Part model, mm, in its own coordinate system. A direction names the side the tool comes from. Give positions to 0.01 mm unless a question says otherwise; leave off trailing zeros. Order: outer loops, then holes, each group sorted by start corner. A loop starts at its lowest first (then second) coordinate and runs counter-clockwise, first axis right, second up. Notation, with made-up numbers: M 89.25,-5 L 130.25,-5 A38 ccw 130.25,34 Z; hole C 10,-32.5 d1. An arc over 180 degrees is marked long. One line per question, with ' | ' between items.
Autodesk Inventor part; units mm, degrees
ref_plane "YZ Plane" through (0, 0, 0) normal (1, 0, 0) x (0, 1, 0)
ref_plane "XZ Plane" through (0, 0, 0) normal (0, 1, 0) x (-1, 0, 0)
ref_plane "XY Plane" through (0, 0, 0) normal (0, 0, 1) x (1, 0, 0)
sketch "스케치1" plane through (0, 0, 0) normal (0, 0, 1) x (1, 0, 0)
  line L0 (-22.5, -10.25) -> (22.5, -10.25)
  line L1 (22.5, -10.25) -> (22.5, 10.25)
  line L2 (22.5, 10.25) -> (-22.5, 10.25)
  line L3 (-22.5, 10.25) -> (-22.5, -10.25)
  line L4 (-22.5, -10.25) -> (22.5, 10.25) construction
  line L5 (22.5, -10.25) -> (-22.5, 10.25) construction
  point P0 (0, 0)
  dimension "d0" = 45
  dimension "d1" = 20.5
extrude "돌출1" add sketch "스케치1" along normal blind 1.2
sketch "스케치2" plane through (-22.5, -10.25, 0) normal (-1, 0, 0) x (0, 0, 1)
  line L0 (1.2, 0) -> (1.2, 20.5)
  line L1 (4.05, 6.65) -> (1.2, 6.65) construction
  line L2 (1.2, 6.65) -> (1.2, 13.85)
  line L3 (1.2, 13.85) -> (4.05, 13.85) construction
  line L4 (4.05, 13.2546) -> (4.05, 7.2454)
  line L5 (4.05, 6.65) -> (1.2, 13.85) construction
  line L6 (1.2, 6.65) -> (4.05, 13.85) construction
  line L7 (1.6136, 13.4226) -> (3.4636, 13.7471)
  line L8 (1.6136, 7.0774) -> (3.4636, 6.7529)
  line L9 (1.2, 12.9301) -> (1.2, 7.5699)
  line L10 (3.85, 7.4835) -> (3.85, 13.0165)
  line L11 (3.2636, 13.509) -> (1.8136, 13.2546)
  line L12 (1.4, 12.7621) -> (1.4, 7.7379)
  line L13 (1.8136, 7.2454) -> (3.2636, 6.991)
  line L14 (2.375, 8.25) -> (2.875, 8.25)
  line L15 (2.875, 8.25) -> (2.875, 12.25)
  line L16 (2.875, 12.25) -> (2.375, 12.25)
  line L17 (2.375, 12.25) -> (2.375, 8.25)
  line L18 (2.375, 8.25) -> (2.875, 12.25) construction
  line L19 (2.875, 8.25) -> (2.375, 12.25) construction
  arc A0 (1.6136, 13.4226) -> (1.2, 12.9301) centre (1.7, 12.9301) ccw
  arc A1 (4.05, 13.2546) -> (3.4636, 13.7471) centre (3.55, 13.2546) ccw
  arc A2 (3.4636, 6.7529) -> (4.05, 7.2454) centre (3.55, 7.2454) ccw
  arc A3 (1.2, 7.5699) -> (1.6136, 7.0774) centre (1.7, 7.5699) ccw
  arc A4 (1.4, 7.7379) -> (1.8136, 7.2454) centre (1.9, 7.7379) ccw
  arc A5 (3.2636, 6.991) -> (3.85, 7.4835) centre (3.35, 7.4835) ccw
  arc A6 (3.85, 13.0165) -> (3.2636, 13.509) centre (3.35, 13.0165) ccw
  arc A7 (1.8136, 13.2546) -> (1.4, 12.7621) centre (1.9, 12.7621) ccw
  point P0 (0, 10.25)
  point P1 (2.625, 10.25)
  point P2 (1.2, 10.25)
  point P3 (1.2, 13.35)
  point P4 (1.2, 7.15)
  dimension "d4" = 2.85
  dimension "d5" = 7.2
  dimension "d6" = 0.5
  dimension "d7" = 0.5
  dimension "d8" = 0.2
  dimension "d9" = 0.5
  dimension "d10" = 4
  dimension "d11" = 0.5
extrude "돌출2" add sketch "스케치2" along normal blind 1 and the other way blind 5
sketch "스케치3" plane through (-17.5, -10.25, 0) normal (1, 0, 0) x (0, 0, -1)
  arc A0 (-4.05, 7.2454) -> (-3.4636, 6.7529) centre (-3.55, 7.2454) ccw
  line L0 (-3.4636, 6.7529) -> (-1.6136, 7.0774)
  arc A1 (-1.6136, 7.0774) -> (-1.2, 7.5699) centre (-1.7, 7.5699) ccw
  line L1 (-1.2, 12.9301) -> (-1.2, 7.5699)
  arc A2 (-1.2, 12.9301) -> (-1.6136, 13.4226) centre (-1.7, 12.9301) ccw
  line L2 (-1.6136, 13.4226) -> (-3.4636, 13.7471)
  arc A3 (-3.4636, 13.7471) -> (-4.05, 13.2546) centre (-3.55, 13.2546) ccw
  line L3 (-4.05, 13.2546) -> (-4.05, 7.2454)
  arc A4 (-3.85, 7.4835) -> (-3.2636, 6.991) centre (-3.35, 7.4835) ccw
  line L4 (-3.85, 7.4835) -> (-3.85, 13.0165)
  arc A5 (-3.2636, 13.509) -> (-3.85, 13.0165) centre (-3.35, 13.0165) ccw
  line L5 (-3.2636, 13.509) -> (-1.8136, 13.2546)
  arc A6 (-1.4, 12.7621) -> (-1.8136, 13.2546) centre (-1.9, 12.7621) ccw
  line L6 (-1.4, 12.7621) -> (-1.4, 7.7379)
  arc A7 (-1.8136, 7.2454) -> (-1.4, 7.7379) centre (-1.9, 7.7379) ccw
  line L7 (-1.8136, 7.2454) -> (-3.2636, 6.991)
  point P0 (0, 10.25)
extrude "돌출3" add sketch "스케치3" against normal blind 1 contours L3 A3 L2 A2 L1 A1 L0 A0 | L4 A5 L5 A6 L6 A7 L7 A4
sketch "스케치4" plane through (0, 0, 1.2) normal (0, 0, 1) x (1, 0, 0)
  line L0 (12.9932, 5.5013) -> (12.9932, -3.185) construction
  line L1 (15.2371, 5.5013) -> (15.2371, -3.185)
  line L2 (10.7492, -3.185) -> (10.7492, 5.5013)
  arc A0 (15.2371, 5.5013) -> (10.7492, 5.5013) centre (12.9932, 5.5013) ccw
  arc A1 (10.7492, -3.185) -> (15.2371, -3.185) centre (12.9932, -3.185) ccw
  point P0 (0, 0)
  point P1 (12.9932, 1.1582)
extrude "돌출4" add sketch "스케치4" along normal blind 2.1
fillet "모깎기1" radius 1 4 edges at (12.9932, 7.7452, 3.3) (10.7492, 1.1582, 3.3) (12.9932, -5.4289, 3.3) (15.2371, 1.1582, 3.3)
properties part number "블루투스 모듈"
1. Tool access for faces 5 (the flat face through (-20.458, -3.333, 2.526)), 6 (the flat face through (-17.5, 0, 3)), 7 (the cylindrical face through (13.04, -5.43, 1.74)), 8 (the flat face through (-22.5, 0, 1)), 9 (the flat face through (-21, 0, 3.85)): list every direction of +Z, -Z, +X, -X, +Y, -Y with a clear straight run to the whole face (end or side of a thin tool).
Worked out:
face 5: -X, -Y | face 6: +Z, +Y, -Y | face 7: +Z, -Y | face 8: -Z, -X, +Y, -Y | face 9: -X
2. Mould opens along Z. For faces 1 (the flat face through (-20.965, 3.134, 2.549)), 2 (the flat face through (-23, 0, 1.2)), 3 (the flat face through (-20.458, 3.333, 2.526)), 4 (the flat face through (10.749, 1, 2)) say: released by +Z, released by -Z, zero draft, split by the parting line, or undercut.
Worked out:
face 1: undercut | face 2: released by -Z | face 3: undercut | face 4: zero draft
3. Probe L1, parallel to Z at x = -15.5, y = -4.5; L2, parallel to X at y = -2.5, z = 3.7; L3, parallel to X at y = 2.75, z = 2.7. List the from-to ranges inside material, lowest first. Write a range as from..to.
Worked out:
L1: z = 0..1.2 | L2: x = -18.5..-17.5 | L3: x = -18.5..-17.5, 10.83..15.15
4. Slice it at B-B on y = 4.5. Give the cut face in (x, z), then the cut area to 3 significant figures.
Worked out:
outline: M -22.5,0 L 22.5,0 L 22.5,1.2 L 15.24,1.2 L 15.24,2.3 A1 ccw 14.24,3.3 L 11.75,3.3 A1 ccw 10.75,2.3 L 10.75,1.2 L -22.5,1.2 Z | area: 63.0 mm2
5. Slice it at C-C on z = 0.7. Give the cut face in (x, y), then the cut area to 4 significant figures.
Worked out:
outline: M -22.5,-10.25 L 22.5,-10.25 L 22.5,10.25 L -22.5,10.25 Z | area: 922.5 mm2
6. Slice it at D-D on x = 6. Give the cut face in (y, z).
Worked out:
outline: M -10.25,0 L 10.25,0 L 10.25,1.2 L -10.25,1.2 Z
7. Drop flat-ended pins along their axis: pin 1 (0.7 mm diameter, centred on x = 12.5, y = -0.5, fed in from +Z); pin 2 (1.2 mm diameter, centred on y = 0.5, z = 2, fed in from +X); pin 3 (3 mm diameter, centred on x = 1.5, y = 6.5, fed in from +Z). Give the stop position or say it passes through.
Worked out:
pin 1: stops at z = 3.3 | pin 2: stops at x = 15.24 | pin 3: stops at z = 1.2
8. Slice it at A-A on x = -19.5. Give the number of separate pieces and of enclosed holes in the cut face, then the cut area to 3 significant figures.
Worked out:
separate pieces: 2 | enclosed holes: 1 | area: 30.3 mm2
